from build123d import *

# Parameters (mm, degrees)
SKETCH_1_W          = 80
SKETCH_1_H          = 27
EXTRUDE_1_DEPTH     = 9.5
SKETCH_3_R          = 7.5
CUT_EXTRUDE_1_DEPTH = 44.272393047
SKETCH_4_R          = 5.15
CUT_EXTRUDE_2_DEPTH = 44.272393047
SKETCH_5_R          = 1.8
CUT_EXTRUDE_3_DEPTH = 44.272393047
SKETCH_7_W          = 1.5
SKETCH_7_H          = 3
CUT_EXTRUDE_4_DEPTH = 44.272393047


with BuildPart() as part:
    # 草图1 → 凸台-拉伸1 (new body)
    with BuildSketch(Plane(origin=(0, 0, 0), x_dir=(1, 0, 0), z_dir=(0, 1, 0))):
        Rectangle(SKETCH_1_W, SKETCH_1_H)
    extrude(amount=EXTRUDE_1_DEPTH)

    # 草图3 → 切除-拉伸1 (cut, through all)
    with BuildSketch(Plane(origin=(0, 9.5, 0), x_dir=(1, 0, 0), z_dir=(0, 1, 0))):
        with Locations(Location((-27, 0, 0), (0, 0, 270))):
            Circle(SKETCH_3_R)
        with Locations(Location((27, 0, 0), (0, 0, 270))):
            Circle(SKETCH_3_R)
    extrude(amount=-CUT_EXTRUDE_1_DEPTH, mode=Mode.SUBTRACT)

    # 草图4 → 切除-拉伸2 (cut, through all)
    with BuildSketch(Plane(origin=(0, 9.5, 0), x_dir=(1, 0, 0), z_dir=(0, 1, 0))):
        with Locations(Location((0, 0, 0), (0, 0, 270))):
            Circle(SKETCH_4_R)
    extrude(amount=-CUT_EXTRUDE_2_DEPTH, mode=Mode.SUBTRACT)

    # 草图5 → 切除-拉伸3 (cut, through all)
    with BuildSketch(Plane(origin=(0, 9.5, 0), x_dir=(1, 0, 0), z_dir=(0, 1, 0))):
        with Locations(Location((8, 0, 0), (0, 0, 270))):
            Circle(SKETCH_5_R)
        with Locations(Location((-8, 0, 0), (0, 0, 270))):
            Circle(SKETCH_5_R)
        with Locations(Location((0, 8, 0), (0, 0, 270))):
            Circle(SKETCH_5_R)
        with Locations(Location((0, -8, 0), (0, 0, 270))):
            Circle(SKETCH_5_R)
    extrude(amount=-CUT_EXTRUDE_3_DEPTH, mode=Mode.SUBTRACT)

    # 草图7 → 切除-拉伸4 (cut, through all)
    with BuildSketch(Plane(origin=(0, 9.5, 0), x_dir=(1, 0, 0), z_dir=(0, 1, 0))):
        with Locations((39.25, 9.501563289)):
            Rectangle(SKETCH_7_W, SKETCH_7_H)
        with Locations((39.25, -9.49986112)):
            Rectangle(SKETCH_7_W, SKETCH_7_H)
        with Locations((-39.25, 9.501563289)):
            Rectangle(SKETCH_7_W, SKETCH_7_H)
        with Locations((-39.25, -9.506798333)):
            Rectangle(SKETCH_7_W, SKETCH_7_H)
    extrude(amount=-CUT_EXTRUDE_4_DEPTH, mode=Mode.SUBTRACT)


solid = part.part
Geometry check sheet. Reference: the model listing, model coordinates, mm. A direction names the side the tool comes from. Give positions to 0.01 mm unless a question says otherwise; leave off trailing zeros. Loops run counter-clockwise (first coordinate to the right, second up) from the corner with the lowest first, then second, coordinate; pieces in that order, holes last. Notation, with made-up numbers: (69.25, 81.5) -> (110.25, 81.5) arc R31 ccw to (110.25, 106.5) -> close; hole circle Ø4 at (67.25, 47.5). An arc over 180 degrees is marked (long way). Answer in a Markdown table with one row per item. Add a question column.
1) Set-up check for faces 5 (the face through (-39, 5, -11.002)), 6 (the face through (39, 5, 11)), 7 (the face through (-40, 5, -12)): record each of +Z, -Z, +X, -X, +Y, -Y from which the full face is reachable in a straight line by a thin tool's end or side.
2) Draft check along X on faces 1 (the face through (-5.028, 4.816, -1.116)), 2 (the face through (40, 5, 12)), 3 (the face through (-9.757, 4.816, -0.39)), 4 (the face through (39, 5, -11.002)). Enter one of: pulls with the +X half, pulls with the -X half, needs draft (parallel to the pull), parting line crosses it, or undercut.
3) Cross-section at A-A on z = 0. Record the boundary of the cut face in (x, y), and give its area (3 significant figures).
4) Cross-section at C-C on y = 1. Record the boundary of the cut face in (x, z), and give its area (3 significant figures).
5) Material ranges on probe 1 along X at (y, z) = (7, 0); probe 2 along X at (y, z) = (7.5, -6.5); probe 3 along X at (y, z) = (3.25, 4), recorded low to high. Write a range as from..to.
6) Cross-section at D-D on x = -8. Record the boundary of the cut face in (y, z), and give its area (3 significant figures).
7) Cross-section at B-B on x = 0. Record the boundary of the cut face in (y, z).
Outcome:
| question | item | result |
|---|---|---|
| 1 | face 5 | -X, +Y, -Y |
| 1 | face 6 | +X, +Y, -Y |
| 1 | face 7 | +Z, -Z, -X, +Y, -Y |
| 2 | face 1 | undercut |
| 2 | face 2 | pulls with the +X half |
| 2 | face 3 | undercut |
| 2 | face 4 | needs draft |
| 3 | outline | (-40, 0) -> (-34.5, 0) -> (-34.5, 9.5) -> (-40, 9.5) -> close; (-19.5, 0) -> (-9.8, 0) -> (-9.8, 9.5) -> (-19.5, 9.5) -> close; (-6.2, 0) -> (-5.15, 0) -> (-5.15, 9.5) -> (-6.2, 9.5) -> close; (5.15, 0) -> (6.2, 0) -> (6.2, 9.5) -> (5.15, 9.5) -> close; (9.8, 0) -> (19.5, 0) -> (19.5, 9.5) -> (9.8, 9.5) -> close; (34.5, 0) -> (40, 0) -> (40, 9.5) -> (34.5, 9.5) -> close |
| 3 | area | 309 mm^2 |
| 4 | outline | (-40, -13.5) -> (40, -13.5) -> (40, -11) -> (38.5, -11) -> (38.5, -8) -> (40, -8) -> (40, 8) -> (38.5, 8) -> (38.5, 11) -> (40, 11) -> (40, 13.5) -> (-40, 13.5) -> (-40, 11.01) -> (-38.5, 11.01) -> (-38.5, 8.01) -> (-40, 8.01) -> (-40, -8) -> (-38.5, -8) -> (-38.5, -11) -> (-40, -11) -> close; hole circle Ø15 at (-27, 0); hole circle Ø3.6 at (-8, 0); hole circle Ø10.3 at (0, 0); hole circle Ø3.6 at (0, -8); hole circle Ø3.6 at (0, 8); hole circle Ø3.6 at (8, 0); hole circle Ø15 at (27, 0) |
| 4 | area | 1,660 mm^2 |
| 5 | probe 1 | x = -40..-34.5, -19.5..-9.8, -6.2..-5.15, 5.15..6.2, 9.8..19.5, 34.5..40 |
| 5 | probe 2 | x = -40..-30.74, -23.26..-0.99, 0.99..23.26, 30.74..40 |
| 5 | probe 3 | x = -40..-33.34, -20.66..-3.24, 3.24..20.66, 33.34..40 |
| 6 | outline | (0, -13.5) -> (9.5, -13.5) -> (9.5, -1.8) -> (0, -1.8) -> close; (0, 1.8) -> (9.5, 1.8) -> (9.5, 13.5) -> (0, 13.5) -> close |
| 6 | area | 222 mm^2 |
| 7 | outline | (0, -13.5) -> (9.5, -13.5) -> (9.5, -9.8) -> (0, -9.8) -> close; (0, -6.2) -> (9.5, -6.2) -> (9.5, -5.15) -> (0, -5.15) -> close; (0, 5.15) -> (9.5, 5.15) -> (9.5, 6.2) -> (0, 6.2) -> close; (0, 9.8) -> (9.5, 9.8) -> (9.5, 13.5) -> (0, 13.5) -> close |
